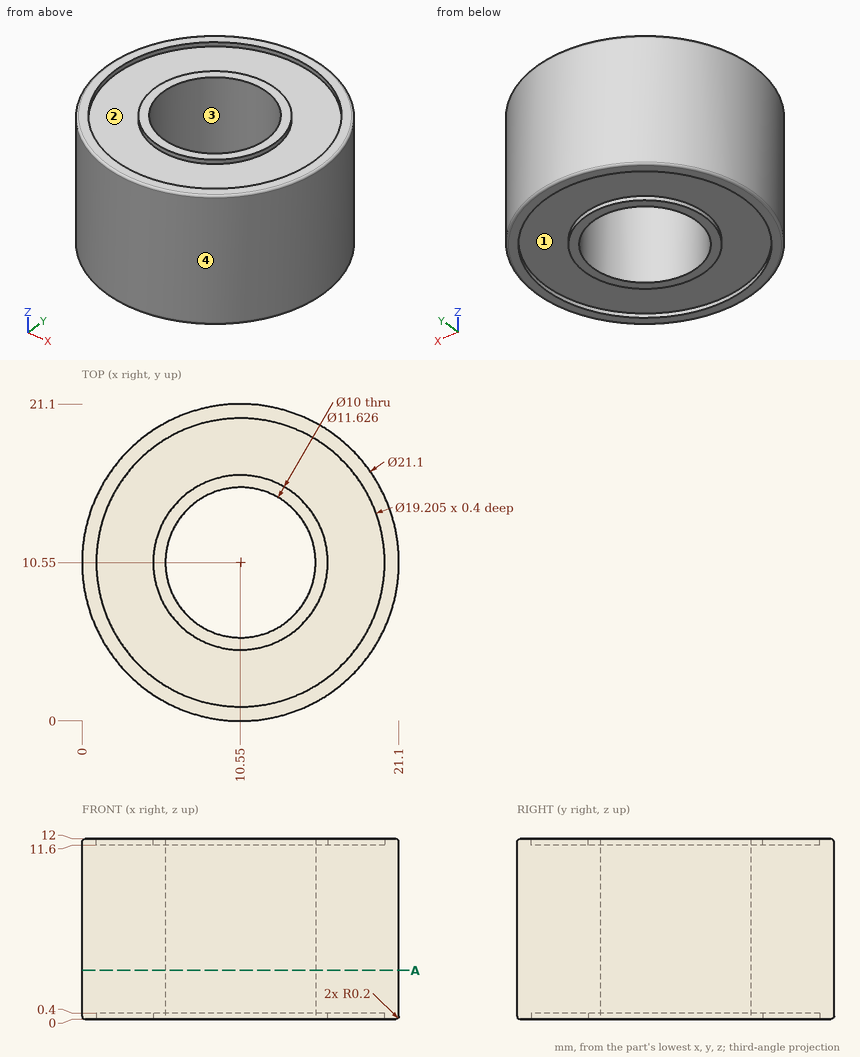
Print and shaded views of the part. All mm, measured from the part's lowest x, y and z. A direction names the side the tool comes from. Coordinates: 2 decimals unless noted, no trailing zeros. Order: outer loops, then holes, each group sorted by start corner. A loop starts at its lowest first (then second) coordinate and runs counter-clockwise, first axis right, second up. Notation, with made-up numbers: (72.5, 88.5) - (108.5, 88.5) arc R21 ccw to (108.5, 107.5) - close; hole circle Ø9 at (-5, -22.75). An arc over 180 degrees is marked (long way). Return JSON: item names as keys, results as strings. Group by question number.
Item 1: Drill centre lines: probe 1 along Y at (x, z) = (10.55, 11.8); probe 2 along Y at (x, z) = (10.55, 3.75); probe 3 along Z at (x, y) = (17.25, 8.75). Where is each one in solid material? Low to high. Write a range as from..to.
Item 2: Cut at A-A (z = 3.25). List the corners of the cut face in (x, y), plus the area to 3 significant figures.
Item 3: Which spindle directions (+Z, -Z, +X, -X, +Y, -Y) get a long thin tool onto all of the face, cutting with end or side? Do the marked faces 1 and 2. Say none if no direction does.
Item 4: Pull direction X, two halves, no side cores. Call the marked faces 3 and 4: pulls with the +X half, pulls with the -X half, needs draft (parallel to the pull), parting line crosses it, or undercut.
Item 5: Pin check, flat tips, straight feed: pin 1 (1.5 mm diameter, centred on y = 13.5, z = 8.5, fed in from -X); pin 2 (2 mm diameter, centred on y = 15.5, z = 5.5, fed in from -X); pin 3 (5 mm diameter, centred on y = 17.5, z = 8.5, fed in from -X) (1 decimal); pin 4 (9 mm diameter, centred on x = 10.55, y = 10.55, fed in from -Z). Stop position of each tip, or through.
Check values:
{
 "1": {"probe 1": "y = 0..0.95, 4.74..5.55, 15.55..16.36, 20.15..21.1", "probe 2": "y = 0..5.55, 15.55..21.1", "probe 3": "z = 0.4..11.6"},
 "2": {"outline": "circle Ø21.1 at (10.55, 10.55); hole circle Ø10 at (10.55, 10.55)", "area": "271 mm2"},
 "3": {"face 1": "-Z", "face 2": "+Z"},
 "4": {"face 3": "undercut", "face 4": "parting line crosses it"},
 "5": {"pin 1": "stops at x = 0.23", "pin 2": "stops at x = 0.77", "pin 3": "stops at x = 1", "pin 4": "passes through"}
}
